```python
from build123d import *

# Parameters (mm, degrees)
F1_DEPTH = 20
F2_R     = 25
F3_R     = 10
F4_R     = 18
F5_DEPTH = 30
F7_D     = 10
F8_D     = 14
F8_DEPTH = 25
F8_TIP   = 4.2060243332


with BuildPart() as f1:
    # F0 (on Front) → F1 (new body)
    with BuildSketch(Plane.XZ):
        Polygon((0, 27.6699295265), (-58.3333333333, 0), (0, -27.6699295265), (58.3333333333, 0), align=None)
    extrude(amount=-F1_DEPTH)

    # F2
    f2_edges = [f1.edges().sort_by_distance(p)[0] for p in [
        (0, 10, -27.66993),
        (0, 10, 27.66993),
    ]]
    fillet(f2_edges, radius=F2_R)

    # F3
    f3_edges = [f1.edges().sort_by_distance(p)[0] for p in [
        (-58.333333, 10, 0),
        (58.333333, 10, 0),
    ]]
    fillet(f3_edges, radius=F3_R)

    # F4 (on face) → F5 (join)
    with BuildSketch(Plane.XZ):
        Circle(F4_R)
    extrude(amount=F5_DEPTH)

    # F7 (through all)
    with Locations(Plane.XZ):
        with Locations((-35, 0), (35, 0)):
            Hole(F7_D / 2)

    # F8
    with Locations(Plane.XZ.offset(30)):
        with Locations((0, 0)):
            Hole(F8_D / 2, depth=F8_DEPTH)
            with Locations((0, 0, -(F8_DEPTH + F8_TIP / 2))):  # 118° drill point
                Cone(0, F8_D / 2, F8_TIP, mode=Mode.SUBTRACT)


solid = f1.part
```
Design review of the part built by this model. Coordinates are the model's own, in mm. A direction names the side the tool comes from. Coordinates: 2 decimals unless noted, no trailing zeros. Loops run counter-clockwise (first coordinate to the right, second up) from the corner with the lowest first, then second, coordinate; pieces in that order, holes last. Notation, with made-up numbers: M 4,-36.75 L 19,-36.75 A11 ccw 19,-21.75 Z; hole C 53.5,21 d10. An arc over 180 degrees is marked long. One line per question, with ' | ' between items.
(1) Machinability: for faces 1 (the face through (-1, 20, 0)), 2 (the face through (-6.466, -17.325, -2.681)), which of the approach directions +Z, -Z, +X, -X, +Y, -Y give a long, thin tool a straight path to every point of the face, cutting with its end or side? Answer none if there is none.
Filled in:
face 1: +Z, -Z, +X, -X, +Y | face 2: -Y
(2) Draft analysis for pull direction Z (two halves, no side actions). For faces 3 (the face through (-30, 10, 0)), 4 (the face through (-25.2, 9.86, -15.717)), 5 (the face through (45, 10, 0)), state which applies: released by +Z, released by -Z, zero draft, split by the parting line, or undercut.
Filled in:
face 3: undercut | face 4: released by -Z | face 5: split by the parting line
(3) We need section A-A (x = 33.5). Give the boundary of the cut face in (y, z), and give its area (3 significant figures).
Filled in:
outline: M 0,-11.78 L 20,-11.78 L 20,-4.77 L 0,-4.77 Z; M 0,4.77 L 20,4.77 L 20,11.78 L 0,11.78 Z | area: 280 mm^2
(4) We need section B-B (y = -23.5). Give the boundary of the cut face in (x, z), and give its area (3 significant figures).
Filled in:
outline: C 0,0 d36; hole C 0,0 d14 | area: 864 mm^2
(5) We need section C-C (z = -2). Count the separate pieces of the cut face and the enclosed holes in it, and give its area (3 significant figures).
Filled in:
separate pieces: 3 | enclosed holes: 0 | area: 2,140 mm^2
(6) Wall thickness on probe 1 along Z at (x, y) = (0, -10.25); probe 2 along X at (y, z) = (15, -2); probe 3 along Y at (x, z) = (24, 5.5): over which ranges is each line inside the solid? List them lowest first.
Filled in:
probe 1: z = -18 to -7, 7 to 18 | probe 2: x = -44.8 to -39.58, -30.42 to 30.42, 39.58 to 44.8 | probe 3: y = 0 to 20
(7) For pin 1 Ø6 at (x, z) = (-35, 0) entering from -Y; pin 2 Ø5 at (x, y) = (32.5, 6.5) entering from +Z; pin 3 Ø5 at (x, y) = (-6.5, -22) entering from +Z; pin 4 Ø4 at (x, y) = (-15.5, -9.5) entering from +Z, all flat-tipped, find the tip position at first contact; note any pin that passes through.
Filled in:
pin 1: passes through | pin 2: stops at z = 13.44 | pin 3: stops at z = 17.55 | pin 4: stops at z = 11.91
(8) We need section D-D (x = -35). Give the boundary of the cut face in (y, z), and give its area (3 significant figures).
Filled in:
outline: M 0,-11.07 L 20,-11.07 L 20,-5 L 0,-5 Z; M 0,5 L 20,5 L 20,11.07 L 0,11.07 Z | area: 243 mm^2
